Could you check a few things on this model? Use its own coordinates, in mm. Coordinates: 2 decimals unless noted, no trailing zeros. Loops run counter-clockwise (first coordinate to the right, second up) from the corner with the lowest first, then second, coordinate; pieces in that order, holes last.
from build123d import *

# Parameters (mm, degrees)
SKETCH1_W           = 546.1
SKETCH1_H           = 457.2
BOSS_EXTRUDE1_DEPTH = 3.175
SKETCH2_R           = 2.54
CUT_EXTRUDE1_DEPTH  = 713.226881425
SKETCH4_W           = 152.4
SKETCH4_H           = 152.4
CUT_EXTRUDE2_DEPTH  = 713.226881425


with BuildPart() as part:
    # Sketch1 → Boss-Extrude1 (new body)
    with BuildSketch(Plane(origin=(0, 0, 0), x_dir=(0, 0, -1), z_dir=(1, 0, 0))):
        with Locations((273.05, 228.6)):
            Rectangle(SKETCH1_W, SKETCH1_H)
    extrude(amount=BOSS_EXTRUDE1_DEPTH)

    # Sketch2 → Cut-Extrude1 (cut, through all)
    with BuildSketch(Plane(origin=(3.175, 0, 0), x_dir=(0, 0, -1), z_dir=(1, 0, 0))):
        with Locations((12.7, 444.5)):
            Circle(SKETCH2_R)
        with Locations((63.5, 444.5)):
            Circle(SKETCH2_R)
        with Locations((114.3, 444.5)):
            Circle(SKETCH2_R)
        with Locations((165.1, 444.5)):
            Circle(SKETCH2_R)
        with Locations((215.9, 444.5)):
            Circle(SKETCH2_R)
        with Locations((12.7, 393.7)):
            Circle(SKETCH2_R)
        with Locations((12.7, 342.9)):
            Circle(SKETCH2_R)
        with Locations((12.7, 292.1)):
            Circle(SKETCH2_R)
        with Locations((12.7, 241.3)):
            Circle(SKETCH2_R)
        with Locations((12.7, 190.5)):
            Circle(SKETCH2_R)
        with Locations((12.7, 139.7)):
            Circle(SKETCH2_R)
        with Locations((12.7, 88.9)):
            Circle(SKETCH2_R)
        with Locations((12.7, 38.1)):
            Circle(SKETCH2_R)
        with Locations(Location((533.4, 38.1, 0), (0, 0, 180))):
            Circle(SKETCH2_R)
        with Locations(Location((533.4, 88.9, 0), (0, 0, 180))):
            Circle(SKETCH2_R)
        with Locations(Location((533.4, 139.7, 0), (0, 0, 180))):
            Circle(SKETCH2_R)
        with Locations(Location((533.4, 190.5, 0), (0, 0, 180))):
            Circle(SKETCH2_R)
        with Locations(Location((533.4, 241.3, 0), (0, 0, 180))):
            Circle(SKETCH2_R)
        with Locations(Location((533.4, 292.1, 0), (0, 0, 180))):
            Circle(SKETCH2_R)
        with Locations(Location((533.4, 342.9, 0), (0, 0, 180))):
            Circle(SKETCH2_R)
        with Locations(Location((533.4, 393.7, 0), (0, 0, 180))):
            Circle(SKETCH2_R)
        with Locations(Location((330.2, 444.5, 0), (0, 0, 180))):
            Circle(SKETCH2_R)
        with Locations(Location((381, 444.5, 0), (0, 0, 180))):
            Circle(SKETCH2_R)
        with Locations(Location((431.8, 444.5, 0), (0, 0, 180))):
            Circle(SKETCH2_R)
        with Locations(Location((482.6, 444.5, 0), (0, 0, 180))):
            Circle(SKETCH2_R)
        with Locations(Location((533.4, 444.5, 0), (0, 0, 180))):
            Circle(SKETCH2_R)
    extrude(amount=-CUT_EXTRUDE1_DEPTH, mode=Mode.SUBTRACT)

    # Sketch4 → Cut-Extrude2 (cut, through all)
    with BuildSketch(Plane(origin=(3.175, 0, 0), x_dir=(0, 0, -1), z_dir=(1, 0, 0))):
        with Locations((76.2, 381)):
            Rectangle(SKETCH4_W, SKETCH4_H)
        with Locations((469.9, 381)):
            Rectangle(SKETCH4_W, SKETCH4_H)
    extrude(amount=-CUT_EXTRUDE2_DEPTH, mode=Mode.SUBTRACT)


solid = part.part
(1) For pin 1 (6.5 mm diameter, centred on y = 292.1, z = -533.4, fed in from +X) (3 decimals); pin 2 (1 mm diameter, centred on x = 1, z = -451.5, fed in from +Y); pin 3 (1.6 mm diameter, centred on x = 1, y = 399, fed in from -Z); pin 4 (1.5 mm diameter, centred on x = 1.5, y = 334, fed in from +Z), each with a flat end and sliding along its axis, tell me the tip position at first contact or that it passes through.
Answers:
pin 1: stops at x = 3.175
pin 2: stops at y = 304.8
pin 3: stops at z = -393.7
pin 4: stops at z = -152.4
(2) Imagine slicing it at B-B, the plane z = -100. Write out the boundary of the cut face in (x, y) (3 decimals), and give its area (3 significant figures).
Answers:
outline: (0, 0) - (3.175, 0) - (3.175, 304.8) - (0, 304.8) - close
area: 968 mm2
(3) I need wall thicknesses on probe 1 along Z at (x, y) = (0.8, 444.5); probe 2 along Z at (x, y) = (2.25, 190.5); probe 3 along Z at (x, y) = (0.4, 138.5). Which ranges of each line are inside material? Lowest first, please.
Answers:
probe 1: z = -393.7 to -383.54, -378.46 to -332.74, -327.66 to -218.44, -213.36 to -167.64, -162.56 to -152.4
probe 2: z = -546.1 to -535.94, -530.86 to -15.24, -10.16 to 0
probe 3: z = -546.1 to -535.64, -531.16 to -14.94, -10.46 to 0
(4) Imagine slicing it at A-A, the plane x = 1.95. State how many separate pieces and enclosed holes the cut face has, and give its area (3 significant figures).
Answers:
separate pieces: 1
enclosed holes: 16
area: 203,000 mm2
